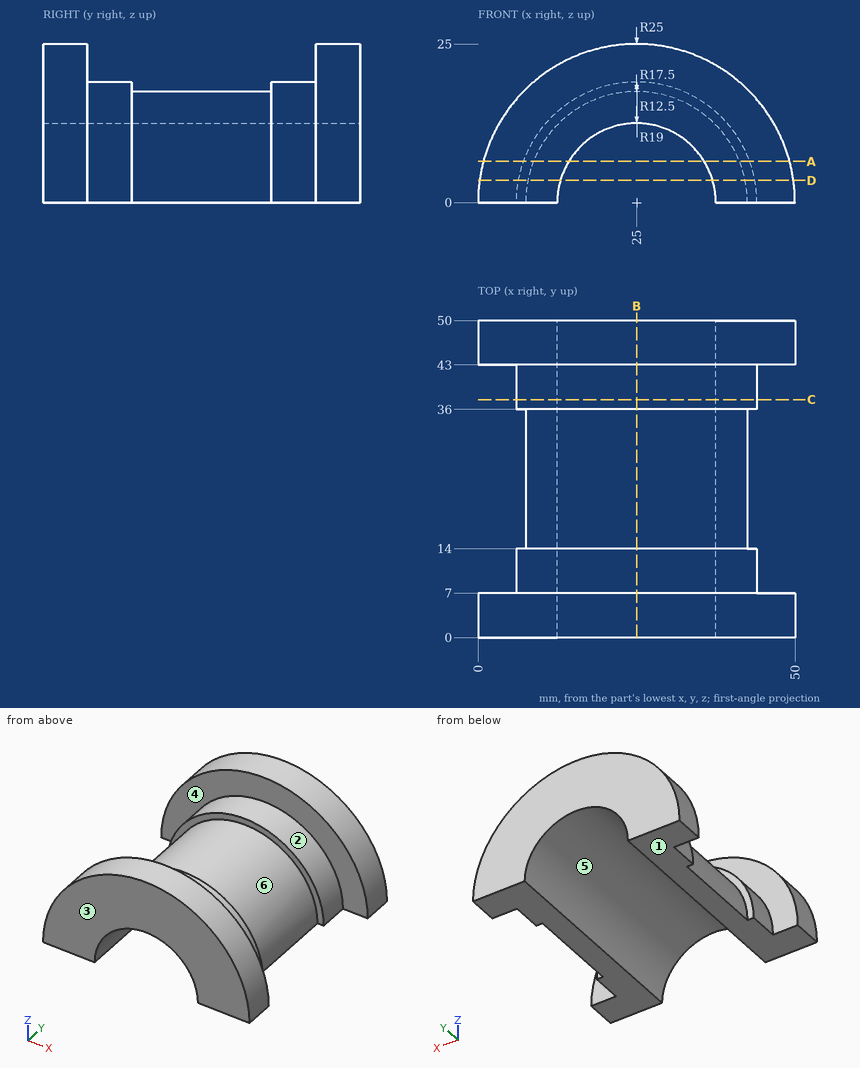
Study the drawing (mm; zero at the part's minimum x, y, z) and answer. A direction names the side the tool comes from. Coordinates: 2 decimals unless noted, no trailing zeros. Write each loop counter-clockwise with the first axis right and the second up, starting at its lowest first coordinate (ties: lowest second). Pieces come first, ordered by that corner, then holes.
Q1. Find the intervals of material crossed by line 1 (Y direction, x = 10.5, z = 15.75); line 2 (Z direction, x = 25.5, y = 27); line 3 (X direction, y = 45, z = 4.75), in increasing order.
Q2. Which of the six approach directions +Z, -Z, +X, -X, +Y, -Y give full straight-line access (tool end or side, diameter ignored) to the marked faces 1 and 2?
Q3. A cutting plane is placed at C-C, the plane y = 37.5. Give the vertices of the cut face in (x, z), then the cut area to 3 significant figures.
Q4. Determine the mould class of the marked faces 3, 4, 5 and 6 for opening direction Y: released by +Y, released by -Y, zero draft, split by the parting line, or undercut.
Q5. A cutting plane is placed at A-A, the plane z = 6.5. Give the vertices of the cut face in (x, y), then the cut area to 3 significant figures.
Q6. Each of these flat-tipped pins is pushed along its axis until it touches: pin 1 Ø4 at (x, y) = (7, 37) entering from +Z; pin 2 Ø8 at (y, z) = (22.5, 18) entering from +X; pin 3 Ø2 at (x, y) = (22, 43.5) entering from +Z. Where does it stop, or does it pass through?
Q7. A cutting plane is placed at D-D, the plane z = 3.5. Give the vertices of the cut face in (x, y), then the cut area to 3 significant figures.
Q8. A cutting plane is placed at B-B, the plane x = 25. Give the vertices of the cut face in (y, z).
Findings below:
1. line 1: y = 0 to 7, 43 to 50
1. line 2: z = 12.49 to 17.49
1. line 3: x = 0.46 to 13.44, 36.56 to 49.54
2. face 1: -Z, +X, -X, +Y, -Y
2. face 2: +Z
3. outline: (6, 0) - (12.5, 0) arc R12.5 cw to (37.5, 0) - (44, 0) arc R19 ccw to start
3. area: 322 mm2
4. face 3: released by -Y
4. face 4: undercut
4. face 5: zero draft
4. face 6: undercut
5. outline: (0.86, 0) - (14.32, 0) - (14.32, 50) - (0.86, 50) - (0.86, 43) - (7.15, 43) - (7.15, 36) - (8.75, 36) - (8.75, 14) - (7.15, 14) - (7.15, 7) - (0.86, 7) - close; (35.68, 0) - (49.14, 0) - (49.14, 7) - (42.85, 7) - (42.85, 14) - (41.25, 14) - (41.25, 36) - (42.85, 36) - (42.85, 43) - (49.14, 43) - (49.14, 50) - (35.68, 50) - close
5. area: 823 mm2
6. pin 1: stops at z = 10.25
6. pin 2: stops at x = 35.5
6. pin 3: stops at z = 24.92
7. outline: (0.25, 0) - (13, 0) - (13, 50) - (0.25, 50) - (0.25, 43) - (6.33, 43) - (6.33, 36) - (7.85, 36) - (7.85, 14) - (6.33, 14) - (6.33, 7) - (0.25, 7) - close; (37, 0) - (49.75, 0) - (49.75, 7) - (43.67, 7) - (43.67, 14) - (42.15, 14) - (42.15, 36) - (43.67, 36) - (43.67, 43) - (49.75, 43) - (49.75, 50) - (37, 50) - close
7. area: 770 mm2
8. outline: (0, 12.5) - (50, 12.5) - (50, 25) - (43, 25) - (43, 19) - (36, 19) - (36, 17.5) - (14, 17.5) - (14, 19) - (7, 19) - (7, 25) - (0, 25) - close
